The model under review builds one solid part; all positions refer to its coordinate system, in mm. A direction names the side the tool comes from. Round coordinates to 2 decimals unless told otherwise and drop trailing zeros. Write each loop counter-clockwise with the first axis right and the second up, starting at its lowest first coordinate (ties: lowest second). Pieces come first, ordered by that corner, then holes. Notation, with made-up numbers: M 68,-8.75 L 72,-8.75 A7 cw 72,-0.75 Z; hole C 87.25,73 d2. An arc over 180 degrees is marked long. Write item = value, one per line. Start each with the question number.
Item 1: Take a section at D-D, the plane z = 0. Give the boundary of the cut face in (x, y).
Item 2: To check wall thickness, follow line 1 along Z through (x, y) = (-15.5, 16); line 2 along Z through (x, y) = (14.5, 28.5); line 3 along X through (y, z) = (4, -16). State the ranges of each line that lie inside material, in increasing order.
Item 3: For pin 1 Ø2 at (x, y) = (-11.5, 20.5) entering from -Z; pin 2 Ø12 at (x, y) = (-2.5, 17) entering from +Z; pin 3 Ø5 at (x, y) = (1.5, 29) entering from -Z, all flat-tipped, find the tip position at first contact; note any pin that passes through.
Item 4: Tool access review of faces 1 (the flat face through (9, 34, 9)), 2 (the flat face through (-6, 2, -23)), 3 (the flat face through (6, 2, -23)), 4 (the flat face through (0, 5, -20)), 5 (the flat face through (0, 17, -19)): name each direction out of +Z, -Z, +X, -X, +Y, -Y from which nothing blocks a thin tool from reaching the whole face with its end or side.
Item 5: Take a section at B-B, the plane x = 0. Give the boundary of the cut face in (y, z).
Item 6: Take a section at C-C, the plane z = -12. Give the boundary of the cut face in (x, y).
Item 7: The part is to be moulded in two halves that separate along Y. For faces 6 (the flat face through (0, 59, 0)), 7 (the flat face through (-17.11, 16.83, -17.06)), 8 (the flat face through (-21, 31, 0)), say which applies: +Y half, -Y half, draft (parallel to the pull), parting line (faces both ways), or undercut.
Item 8: Take a section at A-A, the plane y = 25.5. Give the boundary of the cut face in (x, z).
from build123d import *

# Parameters (mm, degrees)
SKETCH_1_W          = 42
SKETCH_1_H          = 42
EXTRUDE_1_DEPTH     = 34
SKETCH_2_R          = 11
EXTRUDE_2_DEPTH     = 2
SKETCH_3_R          = 3.05
EXTRUDE_3_DEPTH     = 23
SKETCH_4_W          = 6.575865178
SKETCH_4_H          = 2.726578245
CUT_EXTRUDE_1_DEPTH = 18
CUT_EXTRUDE_2_DEPTH = 46.144213361
CHAMFER_1_SIZE      = 5
CUT_EXTRUDE_3_DEPTH = 24
SKETCH_7_W          = 12
SKETCH_7_H          = 5
EXTRUDE_4_DEPTH     = 5
SKETCH_8_W          = 9.77285119
SKETCH_8_H          = 3.692990437
CUT_EXTRUDE_4_DEPTH = 4


with BuildPart() as part:
    # 草图1 → 凸台-拉伸1 (new body)
    with BuildSketch(Plane(origin=(0, 0, 0), x_dir=(1, 0, 0), z_dir=(0, 1, 0))):
        Rectangle(SKETCH_1_W, SKETCH_1_H)
    extrude(amount=EXTRUDE_1_DEPTH)

    # 草图2 → 凸台-拉伸2 (add)
    with BuildSketch(Plane(origin=(0, 34, 0), x_dir=(1, 0, 0), z_dir=(0, 1, 0))):
        with Locations(Location((0, 0, 0), (0, 0, 270))):
            Circle(SKETCH_2_R)
    extrude(amount=EXTRUDE_2_DEPTH)

    # 草图3 → 凸台-拉伸3 (add)
    with BuildSketch(Plane(origin=(0, 36, 0), x_dir=(1, 0, 0), z_dir=(0, 1, 0))):
        with Locations(Location((0, 0, 0), (0, 0, 270))):
            Circle(SKETCH_3_R)
    extrude(amount=EXTRUDE_3_DEPTH)

    # 草图4 → 切除-拉伸1 (cut)
    with BuildSketch(Plane(origin=(0, 59, 0), x_dir=(1, 0, 0), z_dir=(0, 1, 0))):
        with Locations((-0.016038696, 3.672861282)):
            Rectangle(SKETCH_4_W, SKETCH_4_H)
    extrude(amount=-CUT_EXTRUDE_1_DEPTH, mode=Mode.SUBTRACT)

    # 草图5 → 切除-拉伸2 (cut, through all)
    with BuildSketch(Plane(origin=(0, 34, 0), x_dir=(1, 0, 0), z_dir=(0, 1, 0))):
        with BuildLine():
            ThreePointArc((17.1, -15.5), (16.63137085, -14.36862915), (15.5, -13.9))
            Line((15.5, -13.9), (15.5, -15.5))
            Line((15.5, -15.5), (13.9, -15.5))
            ThreePointArc((13.9, -15.5), (15.5, -17.1), (17.1, -15.5))
        make_face()
        with BuildLine():
            Line((15.5, -15.5), (15.5, -13.9))
            ThreePointArc((15.5, -13.9), (14.36862915, -14.36862915), (13.9, -15.5))
            Line((13.9, -15.5), (15.5, -15.5))
        make_face()
        with BuildLine():
            ThreePointArc((-13.9, -15.5), (-14.36862915, -14.36862915), (-15.5, -13.9))
            Line((-15.5, -13.9), (-15.5, -15.5))
            Line((-15.5, -15.5), (-13.9, -15.5))
        make_face()
        with BuildLine():
            Line((-15.5, -15.5), (-15.5, -13.9))
            ThreePointArc((-15.5, -13.9), (-16.63137085, -16.63137085), (-13.9, -15.5))
            Line((-13.9, -15.5), (-15.5, -15.5))
        make_face()
        with BuildLine():
            ThreePointArc((-15.5, 13.9), (-14.36862915, 14.36862915), (-13.9, 15.5))
            Line((-13.9, 15.5), (-15.5, 15.5))
            Line((-15.5, 15.5), (-15.5, 13.9))
        make_face()
        with BuildLine():
            Line((-15.5, 15.5), (-13.9, 15.5))
            ThreePointArc((-13.9, 15.5), (-16.63137085, 16.63137085), (-15.5, 13.9))
            Line((-15.5, 13.9), (-15.5, 15.5))
        make_face()
        with BuildLine():
            ThreePointArc((17.1, 15.5), (15.5, 17.1), (13.9, 15.5))
            Line((13.9, 15.5), (15.5, 15.5))
            Line((15.5, 15.5), (15.5, 13.9))
            ThreePointArc((15.5, 13.9), (16.63137085, 14.36862915), (17.1, 15.5))
        make_face()
        with BuildLine():
            Line((15.5, 15.5), (13.9, 15.5))
            ThreePointArc((13.9, 15.5), (14.36862915, 14.36862915), (15.5, 13.9))
            Line((15.5, 13.9), (15.5, 15.5))
        make_face()
    extrude(amount=-CUT_EXTRUDE_2_DEPTH, mode=Mode.SUBTRACT)

    # 倒角1
    chamfer_1_edges = [part.edges().sort_by_distance(p)[0] for p in [
        (-21, 17, -21),
        (21, 17, -21),
        (21, 17, 21),
        (-21, 17, 21),
    ]]
    chamfer(chamfer_1_edges, length=CHAMFER_1_SIZE)

    # 草图6 → 切除-拉伸3 (cut)
    with BuildSketch(Plane(origin=(0, 5, 0), x_dir=(-1, 0, 0), z_dir=(0, -1, 0))):
        Polygon((-21, 16), (-21, -16), (-16, -21), (16, -21), (21, -16), (21, 16), (16, 21), (-16, 21), align=None)
        Polygon((-19, 15.171572875), (-19, -15.171572875), (-15.171572875, -19), (15.171572875, -19), (19, -15.171572875), (19, 15.171572875), (15.171572875, 19), (-15.171572875, 19), align=None, mode=Mode.SUBTRACT)
    extrude(amount=-CUT_EXTRUDE_3_DEPTH, mode=Mode.SUBTRACT)

    # 草图7 → 凸台-拉伸4 (add)
    with BuildSketch(Plane(origin=(0, 0, -21), x_dir=(-1, 0, 0), z_dir=(0, 0, -1))):
        with Locations((0, 2.5)):
            Rectangle(SKETCH_7_W, SKETCH_7_H)
    extrude(amount=EXTRUDE_4_DEPTH)

    # 草图8 → 切除-拉伸4 (cut)
    with BuildSketch(Plane(origin=(0, 0, -26), x_dir=(-1, 0, 0), z_dir=(0, 0, -1))):
        with Locations((0.097667739, 3.153504782)):
            Rectangle(SKETCH_8_W, SKETCH_8_H)
    extrude(amount=-CUT_EXTRUDE_4_DEPTH, mode=Mode.SUBTRACT)


solid = part.part
Response values:
q1.outline = M -21,0 L 21,0 L 21,5 L 19,5 L 19,29 L 21,29 L 21,34 L 11,34 L 11,36 L 3.05,36 L 3.05,59 L -3.05,59 L -3.05,36 L -11,36 L -11,34 L -21,34 L -21,29 L -19,29 L -19,5 L -21,5 Z
q2.line_1 = -18.67 to -17.1, -13.9 to 13.9, 17.1 to 18.67
q2.line_2 = -19 to -16.75, -14.25 to 14.25, 16.75 to 19
q2.line_3 = -21 to -17.02, -13.98 to 13.98, 17.02 to 21
q3.pin_1 = -19
q3.pin_2 = 19
q3.pin_3 = -21
q4.face_1 = +Y
q4.face_2 = -Z, -X, +Y, -Y
q4.face_3 = -Z, +X, +Y, -Y
q4.face_4 = none
q4.face_5 = -Z, +X, -X
q5.outline = M 0,-26 L 1.31,-26 L 1.31,-22 L 5,-22 L 5,-19 L 29,-19 L 29,-21 L 34,-21 L 34,-11 L 36,-11 L 36,-3.05 L 41,-3.05 L 41,-2.31 L 59,-2.31 L 59,3.05 L 36,3.05 L 36,11 L 34,11 L 34,21 L 29,21 L 29,19 L 5,19 L 5,21 L 0,21 Z
q6.outline = M -21,0 L 21,0 L 21,5 L 19,5 L 19,29 L 21,29 L 21,34 L -21,34 L -21,29 L -19,29 L -19,5 L -21,5 Z
q7.face_6 = +Y half
q7.face_7 = undercut
q7.face_8 = draft
q8.outline = M -19,-15.17 L -15.17,-19 L 15.17,-19 L 19,-15.17 L 19,15.17 L 15.17,19 L -15.17,19 L -19,15.17 Z; hole C -15.5,-15.5 d3.2; hole C -15.5,15.5 d3.2; hole C 15.5,-15.5 d3.2; hole C 15.5,15.5 d3.2
